from build123d import *

# Parameters (mm, degrees)
CROQUIS1_W              = 20
CROQUIS1_H              = 15
CROQUIS1_R              = 1.5
CROQUIS1_R_2            = 2
SALIENTE_EXTRUIR1_DEPTH = 4
CORTAR_EXTRUIR1_DEPTH   = 16


with BuildPart() as part:
    # Croquis1 → Saliente-Extruir1 (new body)
    with BuildSketch(Plane(origin=(0, 0, 0), x_dir=(1, 0, 0), z_dir=(0, 1, 0))):
        Rectangle(CROQUIS1_W, CROQUIS1_H)
        with Locations((-5, 3.75)):
            Circle(CROQUIS1_R, mode=Mode.SUBTRACT)
        with Locations((-5, -3.75)):
            Circle(CROQUIS1_R, mode=Mode.SUBTRACT)
        with Locations((6, 4.5)):
            Circle(CROQUIS1_R_2, mode=Mode.SUBTRACT)
        with Locations((6, -4.5)):
            Circle(CROQUIS1_R_2, mode=Mode.SUBTRACT)
    extrude(amount=SALIENTE_EXTRUIR1_DEPTH)

    # Croquis2 → Cortar-Extruir1 (cut, through all)
    with BuildSketch(Plane(origin=(0, -3.5, 7.5), x_dir=(1, 0, 0), z_dir=(0, 0, -1))):
        Polygon((-10, -7.5), (0, -7.5), (0, -5.5), (-7, -5.5), (-7, -3.5), (-10, -3.5), align=None)
    extrude(amount=CORTAR_EXTRUIR1_DEPTH, mode=Mode.SUBTRACT)


solid = part.part
Input: part model. Units: mm. Frame: model coordinates. A direction names the side the tool comes from. Round coordinates to 2 decimals unless told otherwise and drop trailing zeros. Order: outer loops, then holes, each group sorted by start corner. A loop starts at its lowest first (then second) coordinate and runs counter-clockwise, first axis right, second up.
1. Mould query, pull axis Z, two halves, no side actions, for faces 3 (the face through (3, 2, 7.5)), 4 (the face through (4.4, 2, -3.3)), 5 (the face through (5, 4, 0)). Classes: released by +Z, released by -Z, zero draft, split by the parting line, or undercut.
The answers:
face 3: released by +Z
face 4: undercut
face 5: zero draft
2. Set-up query: faces 1 (the face through (-3, 2, 0)), 2 (the face through (10, 2, 0)). Return all of +Z, -Z, +X, -X, +Y, -Y with unobstructed straight access to the full face (end or side cutting, diameter ignored); none if empty.
The answers:
face 1: +Z, -Z, -X, +Y
face 2: +Z, -Z, +X, +Y, -Y
3. Cut plane A-A, the plane x = -5. Output: boundary loops of the cut face in (y, z), then the cut area to 3 significant figures.
The answers:
outline: (0, -7.5) - (2, -7.5) - (2, -5.25) - (0, -5.25) - close; (0, -2.25) - (2, -2.25) - (2, 2.25) - (0, 2.25) - close; (0, 5.25) - (2, 5.25) - (2, 7.5) - (0, 7.5) - close
area: 18.0 mm2
4. Cut plane D-D, the plane y = 2.85. Output: boundary loops of the cut face in (x, z), then the cut area to 3 significant figures.
The answers:
outline: (0, -7.5) - (10, -7.5) - (10, 7.5) - (0, 7.5) - close; hole circle Ø4 at (6, -4.5); hole circle Ø4 at (6, 4.5)
area: 125 mm2
5. Material intervals for line 1 (Z direction, x = 6, y = 1.3); line 2 (Z direction, x = -5, y = 1.5); line 3 (X direction, y = 1.55, z = 5), sorted ascending.
The answers:
line 1: z = -7.5 to -6.5, -2.5 to 2.5, 6.5 to 7.5
line 2: z = -7.5 to -5.25, -2.25 to 2.25, 5.25 to 7.5
line 3: x = -7 to -5.83, -4.17 to 4.06, 7.94 to 10
6. Cut plane C-C, the plane z = 4.5. Output: boundary loops of the cut face in (x, y).
The answers:
outline: (-7, 0) - (-6.3, 0) - (-6.3, 2) - (-7, 2) - close; (-3.7, 0) - (4, 0) - (4, 4) - (0, 4) - (0, 2) - (-3.7, 2) - close; (8, 0) - (10, 0) - (10, 4) - (8, 4) - close
7. Cut plane B-B, the plane y = 0.9. Output: boundary loops of the cut face in (x, z).
The answers:
outline: (-7, -7.5) - (10, -7.5) - (10, 7.5) - (-7, 7.5) - close; hole circle Ø3 at (-5, -3.75); hole circle Ø3 at (-5, 3.75); hole circle Ø4 at (6, -4.5); hole circle Ø4 at (6, 4.5)
8. Pin query (flat end, axial travel): P1, Ø5, axis at x = -5, z = -3.75, coming from the +Y side; P2, Ø2.5, axis at x = -5, z = 3.75, coming from the -Y side (3 decimals). Return the tip coordinate at first contact, or that it passes through.
The answers:
P1: stops at y = 2
P2: passes through
